Input: part model. Units: mm. Frame: model coordinates. A direction names the side the tool comes from. Coordinates: 2 decimals unless noted, no trailing zeros. Loops run counter-clockwise (first coordinate to the right, second up) from the corner with the lowest first, then second, coordinate; pieces in that order, holes last. Notation, with made-up numbers: (-27.75, -40) - (-20.75, -40) arc R24 cw to (-20.75, -3) - close; hole circle Ø2 at (-31, 66.5). An arc over 180 degrees is marked (long way). Use a Markdown table: item, result. Add a question column.
1. Ray query, L1, parallel to X at y = -12, z = 5.5; L2, parallel to Y at x = 55.5, z = 8.5; L3, parallel to X at y = -29, z = 4. Return the intervals inside material, ascending. Write a range as [from, to].
2. Section query A-A on x = 12.5. Return the cut outline in (y, z).
3. Contact query for flat-ended pins moving along their axis: P1, Ø2, axis at x = -42.5, z = 4.5, coming from the +Y side; P2, Ø3, axis at x = 25, z = 4, coming from the -Y side; P3, Ø6, axis at x = -28, y = 18.5, coming from the +Z side. Output: stop coordinate, or through.
4. Section query C-C on x = 58.5. Return the cut outline in (y, z), then the cut area to 3 significant figures.
5. Section query B-B on y = 39. Return the cut outline in (x, z).
6. Draft query along Y for faces 4 (the face through (-44, -6.664, 6)), 5 (the face through (83.926, -40.161, 6.07)), 6 (the face through (48.926, -11.979, 1.073)), 7 (the face through (83.85, -8.09, 6.07)). Return one class per face: released by +Y, released by -Y, zero draft, split by the parting line, or undercut.
7. Access query for faces 1 (the face through (60.564, 9.322, 1.514)), 2 (the face through (63.062, -32.65, 1.514)), 3 (the face through (14.86, 16.35, 10.486)). Directions: +Z, -Z, +X, -X, +Y, -Y. A direction counts if a zero-diameter tool reaches every point of the face in a straight line with its end or side. Return the directions, or none.
```python
from build123d import *

# Parameters (mm, degrees)
F0_W     = 101
F0_H     = 56
F1_DEPTH = 12
F2_SIZE  = 2.5
F3_R     = 4.99999


# Not quite as in the source:
# - a fillet or chamfer is up to 0.001 mm smaller than in the source, because OpenCascade refuses the exact size


with BuildPart() as f1:
    # F0 (on Top) → F1 (new body)
    with BuildSketch(Plane.XY):
        Polygon((75.1021924019, 82.3358418196), (-43.8978075981, 82.3358418196), (-43.8978075981, 8.3358418196), (-19.1478075981, 8.3358418196), (-9.1478075981, 8.3358418196), (15.6021924019, 8.3358418196), (40.3521924019, 8.3358418196), (50.3521924019, 8.3358418196), (75.1021924019, 8.3358418196), align=None)
        with Locations((15.6021924019, 45.3358418196)):
            Rectangle(F0_W, F0_H, mode=Mode.SUBTRACT)
        Polygon((-9.1478075981, 8.3358418196), (-19.1478075981, 8.3358418196), (-19.1478075981, -31.6641581804), (-44.1478075981, -31.6641581804), (-44.1478075981, -16.6641581804), (-34.1478075981, -16.6641581804), (-34.1478075981, -6.6641581804), (-44.1478075981, -6.6641581804), (-54.1478075981, -6.6641581804), (-54.1478075981, -41.6641581804), (-9.1478075981, -41.6641581804), align=None)
        Polygon((50.3521924019, -31.6641581804), (50.3521924019, 8.3358418196), (40.3521924019, 8.3358418196), (40.3521924019, -41.6641581804), (85.3521924019, -41.6641581804), (85.3521924019, -6.6641581804), (75.3521924019, -6.6641581804), (65.3521924019, -6.6641581804), (65.3521924019, -16.6641581804), (75.3521924019, -16.6641581804), (75.3521924019, -31.6641581804), align=None)
    extrude(amount=F1_DEPTH)

    # F2
    f2_edges = [f1.edges().sort_by_distance(p)[0] for p in [
        (-43.897808, 45.335842, 0),
        (15.602192, 82.335842, 0),
        (75.102192, 45.335842, 0),
        (62.727192, 8.335842, 0),
        (50.352192, -11.664158, 0),
        (62.852192, -31.664158, 0),
        (75.352192, -24.164158, 0),
        (70.352192, -16.664158, 0),
        (65.352192, -11.664158, 0),
        (75.352192, -6.664158, 0),
        (85.352192, -24.164158, 0),
        (62.852192, -41.664158, 0),
        (-31.522808, 8.335842, 0),
        (40.352192, -16.664158, 0),
        (-9.147808, -16.664158, 0),
        (-31.647808, -41.664158, 0),
        (-54.147808, -24.164158, 0),
        (-44.147808, -6.664158, 0),
        (-31.647808, -31.664158, 0),
        (-19.147808, -11.664158, 0),
        (-31.522808, 8.335842, 12),
        (62.727192, 8.335842, 12),
        (15.602192, 82.335842, 12),
        (-43.897808, 45.335842, 12),
        (-19.147808, -11.664158, 12),
        (-31.647808, -31.664158, 12),
        (-44.147808, -24.164158, 12),
        (-39.147808, -16.664158, 12),
        (-34.147808, -11.664158, 12),
        (-44.147808, -6.664158, 12),
        (-54.147808, -24.164158, 12),
        (-31.647808, -41.664158, 12),
        (-9.147808, -16.664158, 12),
        (15.602192, 8.335842, 12),
        (40.352192, -16.664158, 12),
        (62.852192, -41.664158, 12),
        (85.352192, -24.164158, 12),
        (75.352192, -6.664158, 12),
        (65.352192, -11.664158, 12),
        (70.352192, -16.664158, 12),
        (75.352192, -24.164158, 12),
        (62.852192, -31.664158, 12),
        (50.352192, -11.664158, 12),
        (75.102192, 45.335842, 12),
        (15.602192, 17.335842, 12),
        (-34.897808, 45.335842, 12),
        (15.602192, 73.335842, 12),
        (66.102192, 45.335842, 12),
        (-39.147808, -16.664158, 0),
        (-44.147808, -24.164158, 0),
        (-34.147808, -11.664158, 0),
        (15.602192, 8.335842, 0),
    ]]
    chamfer(f2_edges, length=F2_SIZE)

    # F3 (radius 5 in the source; OpenCascade refuses exactly that, so slightly less here)
    f3_edges = [f1.edges().sort_by_distance(p)[0] for p in [
        (-34.897808, 73.335842, 4.75),
        (-34.897808, 17.335842, 4.75),
        (66.102192, 17.335842, 4.75),
        (66.102192, 73.335842, 4.75),
        (75.102192, 8.335842, 6),
        (-43.897808, 8.335842, 6),
        (-43.897808, 82.335842, 6),
        (75.102192, 82.335842, 6),
        (-19.147808, 8.335842, 6),
        (-9.147808, 8.335842, 6),
        (40.352192, 8.335842, 6),
        (50.352192, 8.335842, 6),
        (-9.147808, -41.664158, 6),
        (-54.147808, -41.664158, 6),
        (-54.147808, -6.664158, 6),
        (-34.147808, -6.664158, 6),
        (-34.147808, -16.664158, 6),
        (-44.147808, -16.664158, 6),
        (-44.147808, -31.664158, 6),
        (-19.147808, -31.664158, 6),
        (40.352192, -41.664158, 6),
        (85.352192, -41.664158, 6),
        (85.352192, -6.664158, 6),
        (65.352192, -6.664158, 6),
        (65.352192, -16.664158, 6),
        (75.352192, -16.664158, 6),
        (50.352192, -31.664158, 6),
        (75.352192, -31.664158, 6),
    ]]
    fillet(f3_edges, radius=F3_R)


solid = f1.part
```
Resolved:
| question | item | result |
|---|---|---|
| 1 | L1 | [-54.15, -34.16], [-19.15, -9.15], [40.35, 50.35], [65.36, 85.35] |
| 1 | L2 | [-41.66, -31.66], [8.34, 17.34], [73.34, 82.34] |
| 1 | L3 | [-54.15, -43.57], [-19.73, -9.15], [40.35, 50.93], [74.77, 85.35] |
| 2 | outline | (8.34, 2.5) - (10.84, 0) - (17.34, 0) - (17.34, 9.5) - (14.84, 12) - (10.84, 12) - (8.34, 9.5) - close; (73.34, 0) - (79.84, 0) - (82.34, 2.5) - (82.34, 9.5) - (79.84, 12) - (75.84, 12) - (73.34, 9.5) - close |
| 3 | P1 | y = 81.61 |
| 3 | P2 | y = 8.34 |
| 3 | P3 | z = 11.34 |
| 4 | outline | (-41.66, 2.5) - (-39.16, 0) - (-34.16, 0) - (-31.66, 2.5) - (-31.66, 9.5) - (-34.16, 12) - (-39.16, 12) - (-41.66, 9.5) - close; (8.34, 2.5) - (10.84, 0) - (17.34, 0) - (17.34, 9.5) - (14.84, 12) - (10.84, 12) - (8.34, 9.5) - close; (73.34, 0) - (79.84, 0) - (82.34, 2.5) - (82.34, 9.5) - (79.84, 12) - (75.84, 12) - (73.34, 9.5) - close |
| 4 | area | 305 mm² |
| 5 | outline | (-43.9, 2.5) - (-41.4, 0) - (-34.9, 0) - (-34.9, 9.5) - (-37.4, 12) - (-41.4, 12) - (-43.9, 9.5) - close; (66.1, 0) - (72.6, 0) - (75.1, 2.5) - (75.1, 9.5) - (72.6, 12) - (68.6, 12) - (66.1, 9.5) - close |
| 6 | face 4 | undercut |
| 6 | face 5 | released by -Y |
| 6 | face 6 | undercut |
| 6 | face 7 | released by +Y |
| 7 | face 1 | -Z, +X |
| 7 | face 2 | -Z |
| 7 | face 3 | +Z |
